Could you check a few things on this model? Use its own coordinates, in mm. A direction names the side the tool comes from. Coordinates: 2 decimals unless noted, no trailing zeros. Order: outer loops, then holes, each group sorted by start corner. A loop starts at its lowest first (then second) coordinate and runs counter-clockwise, first axis right, second up. Notation, with made-up numbers: M 53,0.5 L 60,0.5 A16 ccw 60,20.5 Z; hole C -29,-28 d10. An arc over 180 degrees is marked long. Write item = value, one per line. Start each with the question number.
from build123d import *
from OCP.BRepFilletAPI import BRepFilletAPI_MakeChamfer

# Parameters (mm, degrees)
SKETCH1_W                  = 35.58
SKETCH1_H                  = 18
BOSS_EXTRUDE1_DEPTH        = 2.5
CUT_EXTRUDE1_DEPTH         = 2
SKETCH3_W                  = 10.54
SKETCH3_H                  = 1.45
BOSS_EXTRUDE2_DEPTH        = 6.38
CHAMFER1_SIZE              = 6.38
CHAMFER1_SIZE_2            = 2.513148834
SKETCH4_W                  = 3
SKETCH4_H                  = 5.1
CUT_EXTRUDE2_DEPTH         = 6.38
CHAMFER1_OF_MIRROR1_SIZE   = 6.38
CHAMFER1_OF_MIRROR1_SIZE_2 = 2.513148834
SKETCH14_W                 = 1.45
SKETCH14_H                 = 10.54
BOSS_EXTRUDE5_DEPTH        = 6.38
CHAMFER4_SIZE              = 6.38
CHAMFER4_SIZE_2            = 2.513148834
SKETCH15_W                 = 3
SKETCH15_H                 = 5.1
CUT_EXTRUDE4_DEPTH         = 6.38


with BuildPart() as part:
    # Sketch1 → Boss-Extrude1 (new body)
    with BuildSketch(Plane(origin=(0, 0, 0), x_dir=(1, 0, 0), z_dir=(0, 1, 0))):
        with Locations((17.79, 9)):
            Rectangle(SKETCH1_W, SKETCH1_H)
    extrude(amount=BOSS_EXTRUDE1_DEPTH)

    # Sketch2 → Cut-Extrude1 (cut)
    with BuildSketch(Plane(origin=(0, 2.5, 0), x_dir=(1, 0, 0), z_dir=(0, 1, 0))):
        with BuildLine():
            Line((0, 12.03), (30.203676308, 12.03))
            ThreePointArc((30.203676308, 12.03), (33, 8.42), (30.203676308, 4.81))
            Line((30.203676308, 4.81), (0, 4.81))
            Line((0, 4.81), (0, 12.03))
        make_face()
    extrude(amount=-CUT_EXTRUDE1_DEPTH, mode=Mode.SUBTRACT)

    # Sketch3 → Boss-Extrude2 (add)
    with BuildSketch(Plane(origin=(0, 2.5, 0), x_dir=(1, 0, 0), z_dir=(0, 1, 0))):
        with Locations((13, 17.275)):
            Rectangle(SKETCH3_W, SKETCH3_H)
    boss_extrude2 = extrude(amount=BOSS_EXTRUDE2_DEPTH)

    # Chamfer1
    chamfer1_edges_1 = [part.edges().sort_by_distance(p)[0] for p in [
        (18.27, 8.88, -17.275),
    ]]
    chamfer1_side_1 = [part.faces().sort_by_distance(p)[0] for p in [
        (18.27, 8.829737023, -17.275),
    ]]
    chamfer1_edges_2 = [part.edges().sort_by_distance(p)[0] for p in [
        (7.73, 8.88, -17.275),
    ]]
    chamfer1_side_2 = [part.faces().sort_by_distance(p)[0] for p in [
        (7.73, 8.829737023, -17.275),
    ]]
    chamfer1 = BRepFilletAPI_MakeChamfer(part.part.solid().wrapped)
    for e in chamfer1_edges_1:
        chamfer1.Add(CHAMFER1_SIZE - 0.0001, CHAMFER1_SIZE_2 - 0.0001, e.wrapped, chamfer1_side_1[0].wrapped)
    for e in chamfer1_edges_2:
        chamfer1.Add(CHAMFER1_SIZE - 0.0001, CHAMFER1_SIZE_2 - 0.0001, e.wrapped, chamfer1_side_2[0].wrapped)
    add(Compound.cast(chamfer1.Shape()), mode=Mode.REPLACE)  # a hair under: the kernel refuses the full size

    # Sketch4 → Cut-Extrude2 (cut)
    with BuildSketch(Plane.XY.offset(-16.55)):
        with Locations((13, 5.05)):
            Rectangle(SKETCH4_W, SKETCH4_H)
    cut_extrude2 = extrude(amount=-CUT_EXTRUDE2_DEPTH, mode=Mode.SUBTRACT)

    # Mirror1: Boss-Extrude2, Cut-Extrude2 across plane
    add(boss_extrude2.mirror(Plane.XY.offset(-9)))
    add(cut_extrude2.mirror(Plane.XY.offset(-9)), mode=Mode.SUBTRACT)

    # Chamfer1 of Mirror1
    chamfer1_of_mirror1_edges_1 = [part.edges().sort_by_distance(p)[0] for p in [
        (18.27, 8.88, -0.725),
    ]]
    chamfer1_of_mirror1_side_1 = [part.faces().sort_by_distance(p)[0] for p in [
        (18.27, 8.829737023, -0.725),
    ]]
    chamfer1_of_mirror1_edges_2 = [part.edges().sort_by_distance(p)[0] for p in [
        (7.73, 8.88, -0.725),
    ]]
    chamfer1_of_mirror1_side_2 = [part.faces().sort_by_distance(p)[0] for p in [
        (7.73, 8.829737023, -0.725),
    ]]
    chamfer1_of_mirror1 = BRepFilletAPI_MakeChamfer(part.part.solid().wrapped)
    for e in chamfer1_of_mirror1_edges_1:
        chamfer1_of_mirror1.Add(CHAMFER1_OF_MIRROR1_SIZE - 0.0001, CHAMFER1_OF_MIRROR1_SIZE_2 - 0.0001, e.wrapped, chamfer1_of_mirror1_side_1[0].wrapped)
    for e in chamfer1_of_mirror1_edges_2:
        chamfer1_of_mirror1.Add(CHAMFER1_OF_MIRROR1_SIZE - 0.0001, CHAMFER1_OF_MIRROR1_SIZE_2 - 0.0001, e.wrapped, chamfer1_of_mirror1_side_2[0].wrapped)
    add(Compound.cast(chamfer1_of_mirror1.Shape()), mode=Mode.REPLACE)  # a hair under: the kernel refuses the full size

    # Sketch14 → Boss-Extrude5 (add)
    with BuildSketch(Plane(origin=(0, 2.5, 0), x_dir=(1, 0, 0), z_dir=(0, 1, 0))):
        with Locations((34.855, 9.09)):
            Rectangle(SKETCH14_W, SKETCH14_H)
    extrude(amount=BOSS_EXTRUDE5_DEPTH)

    # Chamfer4
    chamfer4_edges_1 = [part.edges().sort_by_distance(p)[0] for p in [
        (34.855, 8.88, -14.36),
    ]]
    chamfer4_side_1 = [part.faces().sort_by_distance(p)[0] for p in [
        (34.855, 8.829737023, -14.36),
    ]]
    chamfer4_edges_2 = [part.edges().sort_by_distance(p)[0] for p in [
        (34.855, 8.88, -3.82),
    ]]
    chamfer4_side_2 = [part.faces().sort_by_distance(p)[0] for p in [
        (34.855, 8.829737023, -3.82),
    ]]
    chamfer4 = BRepFilletAPI_MakeChamfer(part.part.solid().wrapped)
    for e in chamfer4_edges_1:
        chamfer4.Add(CHAMFER4_SIZE - 0.0001, CHAMFER4_SIZE_2 - 0.0001, e.wrapped, chamfer4_side_1[0].wrapped)
    for e in chamfer4_edges_2:
        chamfer4.Add(CHAMFER4_SIZE - 0.0001, CHAMFER4_SIZE_2 - 0.0001, e.wrapped, chamfer4_side_2[0].wrapped)
    add(Compound.cast(chamfer4.Shape()), mode=Mode.REPLACE)  # a hair under: the kernel refuses the full size

    # Sketch15 → Cut-Extrude4 (cut)
    with BuildSketch(Plane.ZY.offset(-34.13)):
        with Locations((-9.09, 5.05)):
            Rectangle(SKETCH15_W, SKETCH15_H)
    extrude(amount=-CUT_EXTRUDE4_DEPTH, mode=Mode.SUBTRACT)


solid = part.part
(1) Imagine slicing it at D-D on z = -2.5. List the corners of the cut face in (x, y) for me.
(2) Imagine slicing it at A-A on x = 6.5. List the corners of the cut face in (y, z) for me, plus the area to 3 significant figures.
(3) Imagine slicing it at C-C on y = 7. List the corners of the cut face in (x, z) for me, plus the area to 3 significant figures.
(4) Please list where these lines run through material, in increasing order: probe 1 along Z at (x, y) = (12, 1.5); probe 2 along Z at (x, y) = (9.5, 4.25); probe 3 along Y at (x, z) = (12, -13). Write a range as from..to.
(5) Thinking about a two-plate mould opening in Z: for faces 4 (the flat face through (16.996, 5.735, -0.735)), 5 (the flat face through (15, 2, -4.81)), 6 (the flat face through (18, 2, 0)), which applies, released by +Z, released by -Z, zero draft, split by the parting line, or undercut?
(6) For faces 1 (the flat face through (17, 0.5, -8)), 2 (the flat face through (35, 7.6, -9)), 3 (the flat face through (14.5, 5, -1)), which set-ups out of +Z, -Z, +X, -X, +Y, -Y let a thin tool reach every point of the face, with its end or its side?
(7) Imagine slicing it at B-B on z = -10. List the corners of the cut face in (x, y) for me, plus the area to 3 significant figures.
(8) Will these pins go through, and if not, where does the flat tip stop? P1, Ø3.5, axis at x = 14, z = -8, coming from the +Y side; P2, Ø9, axis at x = 25.5, z = -7.5, coming from the +Y side; P3, Ø0.7, axis at y = 4, z = -17, coming from the -X side.
Response:
q1.outline = M 0,0 L 35.58,0 L 35.58,2.5 L 0,2.5 Z
q2.outline = M 0,-18 L 2.5,-18 L 2.5,-12.03 L 0.5,-12.03 L 0.5,-4.81 L 2.5,-4.81 L 2.5,0 L 0,0 Z
q2.area = 30.6 mm2
q3.outline = M 9.5,-18 L 11.5,-18 L 11.5,-16.55 L 9.5,-16.55 Z; M 9.5,-1.45 L 11.5,-1.45 L 11.5,0 L 9.5,0 Z; M 14.5,-18 L 16.5,-18 L 16.5,-16.55 L 14.5,-16.55 Z; M 14.5,-1.45 L 16.5,-1.45 L 16.5,0 L 14.5,0 Z; M 34.13,-12.59 L 35.58,-12.59 L 35.58,-10.59 L 34.13,-10.59 Z; M 34.13,-7.59 L 35.58,-7.59 L 35.58,-5.59 L 34.13,-5.59 Z
q3.area = 17.4 mm2
q4.probe_1 = -18..-12.03, -4.81..0
q4.probe_2 = -18..-16.55, -1.45..0
q4.probe_3 = 0..2.5
q5.face_4 = zero draft
q5.face_5 = undercut
q5.face_6 = released by +Z
q6.face_1 = -X, +Y
q6.face_2 = +X, -X
q6.face_3 = +Z, -Z
q7.outline = M 0,0 L 35.58,0 L 35.58,2.5 L 32.65,2.5 L 32.65,0.5 L 0,0.5 Z; M 34.13,7.6 L 35.58,7.6 L 35.58,8.88 L 34.13,8.88 Z
q7.area = 25.5 mm2
q8.P1 = 0.5
q8.P2 = 2.5
q8.P3 = 8.18
